```python
from build123d import *

# Parameters (mm, degrees)
BOX406004_W                 = 5.8
BOX406004_H                 = 14.8
BOX406004_DEPTH             = 2
BOX406004_ROLL_ANGLE        = 89.999938
BOX406004_PITCH_ANGLE       = -2.6e-05
BOX406004_PLACEMENT_ANGLE   = -45.000013
CYLINDER066_R               = 1.75
CYLINDER066_DEPTH           = 33
CYLINDER066_ROLL_ANGLE      = 90.000024
CYLINDER066_PITCH_ANGLE     = 1e-05
CYLINDER066_PLACEMENT_ANGLE = -45.000049
BOX404_W                    = 5
BOX404_H                    = 5
BOX404_DEPTH                = 14
BOX406007_W                 = 14
BOX406007_H                 = 10
BOX406007_DEPTH             = 14
BOX406007_PLACEMENT_ANGLE   = 45
BOX405_W                    = 15
BOX405_H                    = 15
BOX405_DEPTH                = 13
CHAMFER_SIZE                = 8.5
FILLET_R                    = 1.5
BOX406008009_W              = 6
BOX406008009_H              = 6
BOX406008009_DEPTH          = 3
CHAMFER029_SIZE             = 1
CHAMFER030_SIZE             = 1
CHAMFER033_SIZE             = 1
FILLET006_R                 = 3
CHAMFER034_SIZE             = 0.7
CHAMFER042_SIZE             = 0.5


with BuildPart() as box406004:
    # Box406004 → Box406004 (new body)
    with BuildSketch(Plane.XY):
        with Locations((2.9, 7.4)):
            Rectangle(BOX406004_W, BOX406004_H)
    extrude(amount=BOX406004_DEPTH)


with BuildPart() as box406004_1:
    # Box406004 roll: moved
    add(box406004.part.rotate(Axis((0, 0, 0), (1, 0, 0)), BOX406004_ROLL_ANGLE))


with BuildPart() as box406004_2:
    # Box406004 pitch: moved
    add(box406004_1.part.rotate(Axis((0, 0, 0), (0, 1, 0)), BOX406004_PITCH_ANGLE))


with BuildPart() as box406004_3:
    # Box406004 placement: moved
    add(box406004_2.part.moved(Location((15.7, 19.8, 5.1))).rotate(Axis((15.7, 19.8, 5.1), (0, 0, 1)), BOX406004_PLACEMENT_ANGLE))


with BuildPart() as finger_cavity:
    # Cylinder066 → Cylinder066 (new body)
    with BuildSketch(Plane.XY):
        Circle(CYLINDER066_R)
    extrude(amount=CYLINDER066_DEPTH)


with BuildPart() as finger_cavity_1:
    # Cylinder066 roll: moved
    add(finger_cavity.part.rotate(Axis((0, 0, 0), (1, 0, 0)), CYLINDER066_ROLL_ANGLE))


with BuildPart() as finger_cavity_2:
    # Cylinder066 pitch: moved
    add(finger_cavity_1.part.rotate(Axis((0, 0, 0), (0, 1, 0)), CYLINDER066_PITCH_ANGLE))


with BuildPart() as finger_cavity_3:
    # Cylinder066 placement: moved
    add(finger_cavity_2.part.moved(Location((26.8701, 26.8701, 8))).rotate(Axis((26.8701, 26.8701, 8), (0, 0, 1)), CYLINDER066_PLACEMENT_ANGLE))

    # Fusion103077010: union Box406004
    add(box406004_3.part)


with BuildPart() as cube334:
    # Box404 → Box404 (new body)
    with BuildSketch(Plane(origin=(20, 20, -7), x_dir=(1, 0, 0), z_dir=(0, 0, 1))):
        with Locations((2.5, 2.5)):
            Rectangle(BOX404_W, BOX404_H)
    extrude(amount=BOX404_DEPTH)


with BuildPart() as cube338:
    # Box406007 → Box406007 (new body)
    with BuildSketch(Plane.XY):
        with Locations((7, 5)):
            Rectangle(BOX406007_W, BOX406007_H)
    extrude(amount=BOX406007_DEPTH)


with BuildPart() as cube338_1:
    # Box406007 placement: moved
    add(cube338.part.moved(Location((1.78, 11.68, 2))).rotate(Axis((1.78, 11.68, 2), (0, 0, -1)), BOX406007_PLACEMENT_ANGLE))


with BuildPart() as fillet_body:
    # Box405 → Box405 (new body)
    with BuildSketch(Plane(origin=(10, 10, 2), x_dir=(1, 0, 0), z_dir=(0, 0, 1))):
        with Locations((7.5, 7.5)):
            Rectangle(BOX405_W, BOX405_H)
    extrude(amount=BOX405_DEPTH)

    # Chamfer
    chamfer_edges = [fillet_body.edges().sort_by_distance(p)[0] for p in [
        (10, 25, 8.5),
        (25, 10, 8.5),
    ]]
    chamfer(chamfer_edges, length=CHAMFER_SIZE)

    # Cut173011017: cut Cube338
    add(cube338_1.part, mode=Mode.SUBTRACT)

    # Fillet
    fillet_edges = [fillet_body.edges().sort_by_distance(p)[0] for p in [
        (10.551068, 17.051068, 8.5),
        (17.051068, 10.551068, 8.5),
    ]]
    fillet(fillet_edges, radius=FILLET_R)


with BuildPart() as finger:
    # Box406008009 → Box406008009 (new body)
    with BuildSketch(Plane(origin=(19, 19, -7), x_dir=(1, 0, 0), z_dir=(0, 0, 1))):
        with Locations((3, 3)):
            Rectangle(BOX406008009_W, BOX406008009_H)
    extrude(amount=BOX406008009_DEPTH)

    # Chamfer029
    chamfer029_edges = [finger.edges().sort_by_distance(p)[0] for p in [
        (19, 22, -4),
        (22, 19, -4),
    ]]
    chamfer(chamfer029_edges, length=CHAMFER029_SIZE)

    # Chamfer030
    chamfer030_edges = [finger.edges().sort_by_distance(p)[0] for p in [
        (19, 19, -6),
    ]]
    chamfer(chamfer030_edges, length=CHAMFER030_SIZE)

    # Chamfer033
    chamfer033_edges = [finger.edges().sort_by_distance(p)[0] for p in [
        (19, 22.5, -7),
        (19.5, 19.5, -7),
        (22.5, 19, -7),
    ]]
    chamfer(chamfer033_edges, length=CHAMFER033_SIZE)

    # Fusion103077013004017007: union Cube334, Fillet body
    add(cube334.part)
    add(fillet_body.part)

    # Fillet006
    fillet006_edges = [finger.edges().sort_by_distance(p)[0] for p in [
        (25, 25, -5.5),
        (25, 25, -1),
        (25, 25, 4.5),
        (25, 25, 11),
    ]]
    fillet(fillet006_edges, radius=FILLET006_R)

    # Cut173011018: cut finger-cavity
    add(finger_cavity_3.part, mode=Mode.SUBTRACT)

    # Chamfer034
    chamfer034_edges = [finger.edges().sort_by_distance(p)[0] for p in [
        (17.051068, 11.172388, 15),
        (11.611728, 15.990408, 8.5),
        (13.801068, 13.801068, 15),
        (12.56362, 15.038516, 7.999993),
    ]]
    chamfer(chamfer034_edges, length=CHAMFER034_SIZE)

    # Chamfer042
    chamfer042_edges = [finger.edges().sort_by_distance(p)[0] for p in [
        (16.3364, 16.335187, 15),
        (19.094116, 14.991684, 15),
        (17.750614, 17.749401, 15),
        (14.992898, 19.092904, 15),
    ]]
    chamfer(chamfer042_edges, length=CHAMFER042_SIZE)


solid = finger.part
```
Work out the finished part from the listing and answer in its coordinate system (mm). A direction names the side the tool comes from. Give positions to 0.01 mm unless a question says otherwise; leave off trailing zeros. Order: outer loops, then holes, each group sorted by start corner. A loop starts at its lowest first (then second) coordinate and runs counter-clockwise, first axis right, second up. Notation, with made-up numbers: (39.5, 49.25) - (95.5, 49.25) arc R22 cw to (95.5, 61.25) - close; hole circle Ø6 at (-12.5, 36). An arc over 180 degrees is marked (long way). One line per item, written item: value. Start each with the question number.
1. Consider line 1 (Z direction, x = 20.75, y = 19.25); line 2 (Z direction, x = 13.25, y = 18); line 3 (Y direction, x = 19.5, z = 7.25). Determine where each line is inside the solid, lowest interval first.
2. Section A-A, the plane z = 2.25 is taken. Write down the section's boundary in (x, y).
3. Section C-C, the plane z = -5.5 is taken. Write down the section's boundary in (x, y), then the cut area to 3 significant figures.
4. For a pull along X with two mould halves and no side action, classify faces 4 (the face through (19.1, 15, 9.7)), 5 (the face through (17.068, 11.172, 8.064)), 6 (the face through (20, 20, 15)), 7 (the face through (19, 22.5, -5.5)) as released by +X, released by -X, zero draft, split by the parting line, or undercut.
5. Section B-B, the plane z = 11 is taken. Write down the section's boundary in (x, y), then the cut area to 3 significant figures.
6. Which of the six approach directions +Z, -Z, +X, -X, +Y, -Y give full straight-line access (tool end or side, diameter ignored) to faces 1 (the face through (15, 19.1, 9.7)), 2 (the face through (22.5, 19, -5.5)), 3 (the face through (18, 18, 2))?
7. Each of these flat-tipped pins is pushed along its axis until it touches: pin 1 Ø8 at (y, z) = (13, -3.5) entering from +X; pin 2 Ø1.5 at (y, z) = (22, -2) entering from -X; pin 3 Ø1.1 at (x, z) = (23.5, -5.5) entering from -Y. Where does it stop, or does it pass through?
Filled sheet:
1. line 1: -6.25 to -4.75, 2 to 6.61, 9.39 to 15
1. line 2: 2 to 15
1. line 3: 13 to 15.4, 16 to 17.26, 21.74 to 25
2. outline: (11.61, 15.99) - (15.99, 11.61) arc R1.5 ccw to (18.11, 11.61) - (25, 18.5) - (25, 22) arc R3 ccw to (22, 25) - (18.5, 25) - (11.61, 18.11) arc R1.5 ccw to start
3. outline: (19, 20) - (20, 19) - (25, 19) - (25, 22) arc R3 ccw to (22, 25) - (19, 25) - close
3. area: 33.6 mm²
4. face 4: undercut
4. face 5: split by the parting line
4. face 6: zero draft
4. face 7: released by -X
5. outline: (11.61, 15.99) - (15.99, 11.61) arc R1.5 ccw to (18.11, 11.61) - (25, 18.5) - (25, 22) arc R3 ccw to (22, 25) - (18.5, 25) - (11.61, 18.11) arc R1.5 ccw to start; hole (14.29, 18.39) - (18.39, 14.28) - (19.8, 15.7) - (15.7, 19.8) - close
5. area: 110 mm²
6. face 1: +Z
6. face 2: -Z, +X, -X, -Y
6. face 3: -X, -Y
7. pin 1: through
7. pin 2: x = 20
7. pin 3: y = 19
